from build123d import *

# Parameters (mm, degrees)
CUT_EXTRUDE1_DEPTH = 1.04


with BuildPart() as part:
    # Sketch1 → Revolve1 (revolve)
    with BuildSketch(Plane(origin=(0, 0, 0), x_dir=(0, 0, -1), z_dir=(1, 0, 0)), mode=Mode.PRIVATE) as revolve1_sk:
        with BuildLine():
            Line((-1.65, 0), (-1.65, 1.25))
            ThreePointArc((-1.65, 1.25), (-1.293908806, 2.271383865), (-0.38, 2.85))
            Line((-0.38, 2.85), (0, 2.85))
            Line((0, 2.85), (0, 1.5))
            Line((0, 1.5), (8, 1.5))
            Line((8, 1.5), (8, 0))
            Line((8, 0), (-1.65, 0))
        make_face()
    revolve(revolve1_sk.sketch.rotate(Axis((0, 0, 5.584882278), (0, 0, -1)), 180), axis=Axis((0, 0, 5.584882278), (0, 0, -1)))

    # Sketch2 → Cut-Extrude1 (cut)
    with BuildSketch(Plane.XY.offset(1.65)):
        Polygon((0.577350269, -1), (1.154700538, 0), (0.577350269, 1), (-0.577350269, 1), (-1.154700538, 0), (-0.577350269, -1), align=None)
    extrude(amount=-CUT_EXTRUDE1_DEPTH, mode=Mode.SUBTRACT)


solid = part.part
Geometry: final body of the model. Coordinates: model frame, mm. A direction names the side the tool comes from. Round coordinates to 2 decimals unless told otherwise and drop trailing zeros. Loops run counter-clockwise (first coordinate to the right, second up) from the corner with the lowest first, then second, coordinate; pieces in that order, holes last. Notation, with made-up numbers: M 68.25,-14.5 L 112.25,-14.5 A12 ccw 112.25,-0.5 Z; hole C 48.25,-11 d7. An arc over 180 degrees is marked long. Put each result on its own line as item: value. Start each with the question number.
(1) Set-up query: faces 1 (the face through (0, 0, -8)), 2 (the face through (-0.45, -1.43, -4.06)), 3 (the face through (0, -1, 1)). Return all of +Z, -Z, +X, -X, +Y, -Y with unobstructed straight access to the full face (end or side cutting, diameter ignored); none if empty.
(2) Material intervals for line 1 along Z through (x, y) = (-0.45, 0); line 2 along Z through (x, y) = (-1.85, -1.4); line 3 along X through (y, z) = (-0.55, 0.75), sorted ascending. Write a range as [from, to].
(3) Section query A-A (z = -0.25). Return loops of the section in (x, y), then the cut area to 3 significant figures.
(4) Contact query for flat-ended pins moving along their axis: pin 1 Ø1.5 at (y, z) = (2, -2) entering from -X; pin 2 Ø2 at (x, z) = (1.5, -2.5) entering from +Y; pin 3 Ø1 at (x, z) = (-0.5, -6) entering from +Y. Output: stop coordinate, or through.
(5) Draft query along Y for faces 4 (the face through (2.78, 0.62, 0.19)), 5 (the face through (1.2, -1.2, 0)), 6 (the face through (0, 0, 0.61)). Return one class per face: +Y half, -Y half, draft (parallel to the pull), parting line (faces both ways), or undercut.
Findings below:
1. face 1: -Z, +X, -X, +Y, -Y
1. face 2: -Z
1. face 3: +Z
2. line 1: z = [-8, 0.61]
2. line 2: z = [0, 1.25]
2. line 3: x = [-2.66, -0.84], [0.84, 2.66]
3. outline: C 0,0 d3
3. area: 7.07 mm2
4. pin 1: stops at x = -0.83
4. pin 2: stops at y = 1.41
4. pin 3: stops at y = 1.5
5. face 4: parting line
5. face 5: draft
5. face 6: undercut
